Autodesk Inventor part; units mm, degrees
ref_plane "Work Plane3" through (0, 15.875, 0) normal (0, 1, 0) x (1, 0, 0)
ref_plane "YZ Plane" through (0, 0, 0) normal (1, 0, 0) x (0, 1, 0)
ref_plane "XZ Plane" through (0, 0, 0) normal (0, 1, 0) x (-1, 0, 0)
sketch "Sketch1" plane through (0, 0, 0) normal (1, 0, 0) x (0, 1, 0)
  line L0 (0, 0) -> (31.75, 0)
  line L1 (31.75, 0) -> (31.75, -12.7)
  line L2 (31.75, -12.7) -> (0, -12.7)
  line L3 (0, -12.7) -> (0, 0)
  line L4 (28.575, 0) -> (25.4, 0)
  line L5 (25.4, 0) -> (25.4, -12.7)
  line L6 (25.4, -12.7) -> (28.575, -12.7)
  line L7 (28.575, -12.7) -> (28.575, 0)
  dimension "d0" = 31.75
  dimension "d1" = 12.7
  dimension "d4" = 3.175
  dimension "d5" = 12.7
  dimension "d6" = 3.175
extrude "Extrusion1" add sketch "Sketch1" along normal blind 6.35
extrude "Extrusion2" add sketch "Sketch1" against normal blind 1.5875 contours L0 L7 L2 L5
sketch "Sketch2" plane through (-1.5875, 0, 0) normal (-1, 0, 0) x (0, 0, 1)
  line L0 (-12.7, 34.671) -> (0, 34.671)
  line L1 (0, 34.671) -> (0, 19.304)
  line L2 (0, 19.304) -> (-12.7, 19.304)
  line L3 (-12.7, 19.304) -> (-12.7, 34.671)
  line L4 (-12.7, 31.75) -> (-12.7, 28.575)
  line L5 (-12.7, 25.4) -> (0, 25.4)
  line L6 (0, 28.575) -> (-12.7, 28.575)
  point P0 (0, 0)
  dimension "d9" = 12.7
  dimension "d10" = 0
  dimension "d11" = 6.096
  dimension "d12" = 6.096
extrude "Extrusion3" add sketch "Sketch2" along normal blind 3.175
sketch "Sketch3" plane through (0, 0, 0) normal (0, 0, 1) x (1, 0, 0)
  line L0 (-4.7625, 34.671) -> (-4.7625, 31.496)
  line L1 (-4.7625, 19.304) -> (-4.7625, 34.671)
  line L2 (-1.5875, 34.671) -> (-1.5875, 28.575)
  line L3 (-1.5875, 34.671) -> (-3.1623, 34.671)
  line L4 (-1.5875, 34.671) -> (-4.7625, 34.671)
  line L5 (-1.5875, 19.304) -> (-3.1623, 19.304)
  line L6 (-1.5875, 19.304) -> (-4.7625, 19.304)
  line L7 (-4.7625, 19.304) -> (-4.7625, 22.479)
  line L8 (-4.7625, 22.479) -> (-3.1623, 19.304)
  line L9 (-4.7625, 19.304) -> (-3.1623, 19.304)
  line L10 (-4.7625, 31.496) -> (-3.1623, 34.671)
  line L11 (-4.7625, 34.671) -> (-3.1623, 34.671)
  point P0 (0, 0)
  dimension "d16" = 3.175
  dimension "d17" = 1.5748
  dimension "d18" = 1.5748
  dimension "d19" = 3.175
extrude "Extrusion4" cut sketch "Sketch3" against normal through all
ref_plane "Work Plane3" through (0, 15.875, 0) normal (0, 1, 0) x (1, 0, 0)
mirror "Mirror1" about plane through (0, 15.875, 0) normal (0, 1, 0) of "Extrusion2", "Extrusion3", "Extrusion4"
equation "\"d5\" = d1"
equation "\"d9\" = d1"
properties part number "2020liftconecter"
The listing builds one solid part. Answer for the finished solid, in the listing's coordinates (mm). A direction names the side the tool comes from. Coordinates: 2 decimals unless noted, no trailing zeros. Order: outer loops, then holes, each group sorted by start corner. A loop starts at its lowest first (then second) coordinate and runs counter-clockwise, first axis right, second up. Notation, with made-up numbers: (13.25, -17) -> (28.25, -17) arc R20 ccw to (28.25, -13) -> close; hole circle Ø2 at (-19.5, -30.75). An arc over 180 degrees is marked (long way). Answer in a Markdown table with one row per item. Add a question column.
Item 1: Determine the mould class of faces 6 (the face through (-3.95, -1.36, -6.26)), 7 (the face through (-3.95, 10.88, -6.26)), 8 (the face through (-4.762, 27, -6)) for opening direction Y: +Y half, -Y half, draft (parallel to the pull), parting line (faces both ways), or undercut.
Item 2: Each of these flat-tipped pins is pushed along its axis until it touches: P1, Ø1.3, axis at x = -0.5, z = -5.5, coming from the -Y side; P2, Ø5, axis at x = 3, z = -2, coming from the +Y side; P3, Ø0.5, axis at x = -1, z = -7.5, coming from the -Y side (3 decimals). Where does it stop, or does it pass through?
Item 3: Find the intervals of material crossed by L1, parallel to X at y = 31.5, z = -3.5; L2, parallel to Y at x = -1.75, z = -6.75; L3, parallel to Y at x = -1, z = -10 (3 decimals), in increasing order. Write a range as from..to.
Item 4: Find section B-B (x = -2.5). Write down the section's boundary in (y, z), then the cut area to 3 significant figures.
Item 5: Find section A-A (y = 24). Write down the section's boundary in (x, z), then the cut area to 3 significant figures.
Item 6: Find section D-D (x = 2.25). Write down the section's boundary in (y, z), then the cut area to 3 significant figures.
Item 7: Which of the six approach directions +Z, -Z, +X, -X, +Y, -Y give full straight-line access (tool end or side, diameter ignored) to faces 1 (the face through (0, 30, -6)), 2 (the face through (0, 16, -6)), 3 (the face through (-2, 19.304, -6)), 4 (the face through (-1.588, 0, -6)), 5 (the face through (3, 0, -6))?
Result set:
| question | item | result |
|---|---|---|
| 1 | face 6 | -Y half |
| 1 | face 7 | undercut |
| 1 | face 8 | draft |
| 2 | P1 | stops at y = 0 |
| 2 | P2 | stops at y = 31.75 |
| 2 | P3 | stops at y = 3.175 |
| 3 | L1 | x = -4.76..-1.59, 0..6.35 |
| 3 | L2 | y = -2.92..12.45, 19.3..34.67 |
| 3 | L3 | y = 3.175..6.35, 25.4..28.575 |
| 4 | outline | (-2.92, -12.7) -> (12.45, -12.7) -> (12.45, 0) -> (-2.92, 0) -> close; (19.3, -12.7) -> (34.67, -12.7) -> (34.67, 0) -> (19.3, 0) -> close |
| 4 | area | 390 mm² |
| 5 | outline | (-4.76, -12.7) -> (-1.59, -12.7) -> (-1.59, 0) -> (-4.76, 0) -> close; (0, -12.7) -> (6.35, -12.7) -> (6.35, 0) -> (0, 0) -> close |
| 5 | area | 121 mm² |
| 6 | outline | (0, -12.7) -> (31.75, -12.7) -> (31.75, 0) -> (0, 0) -> close |
| 6 | area | 403 mm² |
| 7 | face 1 | +Z, -Z, +Y |
| 7 | face 2 | +Z, -Z |
| 7 | face 3 | +Z, -Z, -X |
| 7 | face 4 | +Z, -Z, -Y |
| 7 | face 5 | +Z, -Z, +X, -Y |
